Input: part model. Units: mm. Frame: model coordinates. Coordinates: 2 decimals unless noted, no trailing zeros. Order: outer loops, then holes, each group sorted by start corner. A loop starts at its lowest first (then second) coordinate and runs counter-clockwise, first axis right, second up. Notation, with made-up numbers: (30, -35) - (67, -35) arc R15 cw to (67, -19) - close; hole circle Ø8 at (70.5, 12). An arc over 180 degrees is marked (long way). Answer as CSV lines item,"result". Start each with the question number.
Item 1: First-contact query: pin 1 (5.5 mm diameter, centred on x = 99.5, y = 80, fed in from -Z); pin 2 (3 mm diameter, centred on x = 20.5, y = 80, fed in from +Z); pin 3 (0.9 mm diameter, centred on x = 11, y = 28, fed in from +Z). Flat tips, straight axial feed; report the tip coordinate or a pass-through.
Item 2: Material intervals for line 1 along X through (y, z) = (80, 2.5); line 2 along Y through (x, z) = (99.5, 2.85); line 3 along X through (y, z) = (69.5, 4.8), sorted ascending.
Item 3: Section A-A (z = 4.2). Output: boundary loops of the cut face in (x, y).
Item 4: Section D-D (x = 55.5). Output: boundary loops of the cut face in (y, z), and give its area (3 significant figures).
Item 5: Section B-B (x = 99.5). Output: boundary loops of the cut face in (y, z), and give its area (3 significant figures).
Item 6: Section C-C (y = 61). Output: boundary loops of the cut face in (x, z).
from build123d import *

# Parameters (mm, degrees)
SKETCH_1_W          = 120
SKETCH_1_H          = 100
SKETCH_1_R          = 1.75
SKETCH_1_W_2        = 65
SKETCH_1_H_2        = 84
EXTRUDE_1_DEPTH     = 5
SKETCH_2_W          = 3
SKETCH_2_H          = 100
CUT_EXTRUDE_1_DEPTH = 2


with BuildPart() as part:
    # 草图1 → 凸台-拉伸1 (new body)
    with BuildSketch(Plane.XY):
        with Locations((60, 50)):
            Rectangle(SKETCH_1_W, SKETCH_1_H)
        with Locations((20.5, 80)):
            Circle(SKETCH_1_R, mode=Mode.SUBTRACT)
        with Locations((20.5, 61)):
            Circle(SKETCH_1_R, mode=Mode.SUBTRACT)
        with Locations((99.5, 80)):
            Circle(SKETCH_1_R, mode=Mode.SUBTRACT)
        with Locations((99.5, 61)):
            Circle(SKETCH_1_R, mode=Mode.SUBTRACT)
        with Locations((60, 50)):
            Rectangle(SKETCH_1_W_2, SKETCH_1_H_2, mode=Mode.SUBTRACT)
    extrude(amount=EXTRUDE_1_DEPTH)

    # 草图2 → 切除-拉伸1 (cut)
    with BuildSketch(Plane.XY.offset(5)):
        with Locations((10.45, 50)):
            Rectangle(SKETCH_2_W, SKETCH_2_H)
        with Locations((109.55, 50)):
            Rectangle(SKETCH_2_W, SKETCH_2_H)
    extrude(amount=-CUT_EXTRUDE_1_DEPTH, mode=Mode.SUBTRACT)


solid = part.part
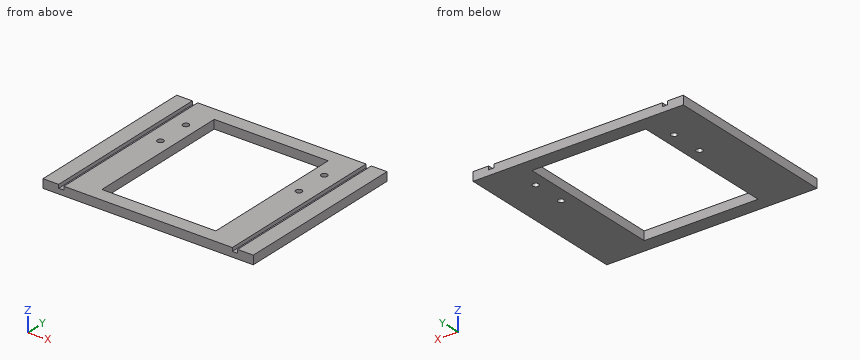
Determined:
1,pin 1,"stops at z = 0"
1,pin 2,"passes through"
1,pin 3,"stops at z = 3"
2,line 1,"x = 0 to 18.75, 22.25 to 27.5, 92.5 to 97.75, 101.25 to 120"
2,line 2,"y = 0 to 59.25, 62.75 to 78.25, 81.75 to 100"
2,line 3,"x = 0 to 8.95, 11.95 to 27.5, 92.5 to 108.05, 111.05 to 120"
3,outline,"(0, 0) - (8.95, 0) - (8.95, 100) - (0, 100) - close; (11.95, 0) - (108.05, 0) - (108.05, 100) - (11.95, 100) - close; (111.05, 0) - (120, 0) - (120, 100) - (111.05, 100) - close; hole circle Ø3.5 at (20.5, 61); hole circle Ø3.5 at (20.5, 80); hole (27.5, 8) - (92.5, 8) - (92.5, 92) - (27.5, 92) - close; hole circle Ø3.5 at (99.5, 61); hole circle Ø3.5 at (99.5, 80)"
4,outline,"(0, 0) - (8, 0) - (8, 5) - (0, 5) - close; (92, 0) - (100, 0) - (100, 5) - (92, 5) - close"
4,area,"80.0 mm^2"
5,outline,"(0, 0) - (59.25, 0) - (59.25, 5) - (0, 5) - close; (62.75, 0) - (78.25, 0) - (78.25, 5) - (62.75, 5) - close; (81.75, 0) - (100, 0) - (100, 5) - (81.75, 5) - close"
5,area,"465 mm^2"
6,outline,"(0, 0) - (18.75, 0) - (18.75, 5) - (11.95, 5) - (11.95, 3) - (8.95, 3) - (8.95, 5) - (0, 5) - close; (22.25, 0) - (27.5, 0) - (27.5, 5) - (22.25, 5) - close; (92.5, 0) - (97.75, 0) - (97.75, 5) - (92.5, 5) - close; (101.25, 0) - (120, 0) - (120, 5) - (111.05, 5) - (111.05, 3) - (108.05, 3) - (108.05, 5) - (101.25, 5) - close"
